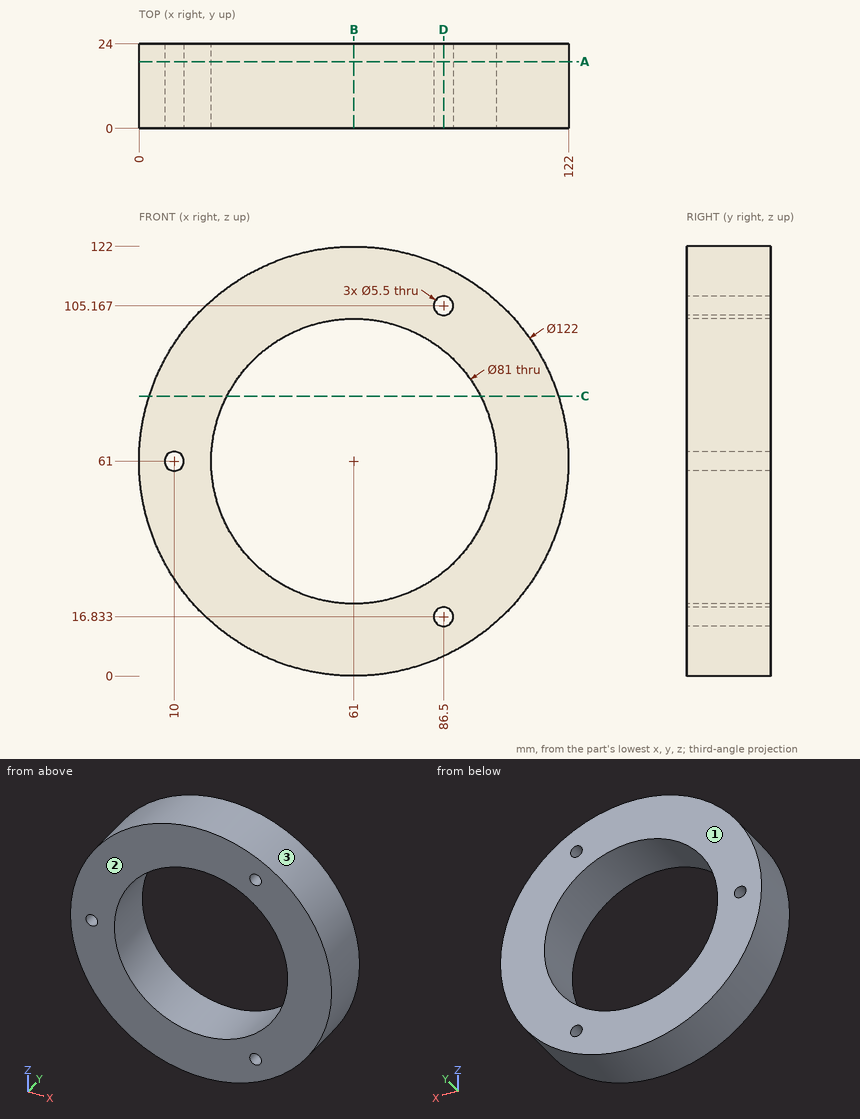
Study the drawing (mm; zero at the part's minimum x, y, z) and answer. Round coordinates to 2 decimals unless told otherwise and drop trailing zeros. Loops run counter-clockwise (first coordinate to the right, second up) from the corner with the lowest first, then second, coordinate; pieces in that order, holes last.
Q1. Given pin 1 Ø1.5 at (x, y) = (14, 12.5) entering from -Z; pin 2 Ø3 at (y, z) = (4.5, 54.5) entering from +X (1 decimal); pin 3 Ø6 at (y, z) = (3.5, 24.5) entering from +X; pin 4 Ø3.5 at (x, z) = (86.5, 16.83) entering from +Y, each flat-ended and moving along its own axis, determine where each tip first touches the part or whether it passes through.
Q2. Section B-B, the plane x = 61 is taken. Determine the outline of the cut face in (y, z), then the cut area to 3 significant figures.
Q3. Section D-D, the plane x = 86.5 is taken. Determine the outline of the cut face in (y, z).
Q4. Find the intervals of material crossed by line 1 (Z direction, x = 60.5, y = 4.5); line 2 (Z direction, x = 86.5, y = 6) (1 decimal); line 3 (Z direction, x = 40.5, y = 6.25), in increasing order.
Q5. For a pull along Y with two mould halves and no side action, classify the marked faces 1, 2 and 3 as released by +Y, released by -Y, zero draft, split by the parting line, or undercut.
Q6. Section A-A, the plane y = 19 is taken. Determine the outline of the cut face in (x, z).
Q7. Section C-C, the plane z = 79.5 is taken. Determine the outline of the cut face in (x, y).
Completed:
1. pin 1: stops at z = 21.23
1. pin 2: stops at x = 121.8
1. pin 3: stops at x = 111.98
1. pin 4: passes through
2. outline: (0, 0) - (24, 0) - (24, 20.5) - (0, 20.5) - close; (0, 101.5) - (24, 101.5) - (24, 122) - (0, 122) - close
2. area: 984 mm2
3. outline: (0, 5.59) - (24, 5.59) - (24, 14.08) - (0, 14.08) - close; (0, 19.58) - (24, 19.58) - (24, 29.54) - (0, 29.54) - close; (0, 92.46) - (24, 92.46) - (24, 102.42) - (0, 102.42) - close; (0, 107.92) - (24, 107.92) - (24, 116.41) - (0, 116.41) - close
4. line 1: z = 0 to 20.5, 101.5 to 122
4. line 2: z = 5.6 to 14.1, 19.6 to 29.5, 92.5 to 102.4, 107.9 to 116.4
4. line 3: z = 3.55 to 26.07, 95.93 to 118.45
5. face 1: released by +Y
5. face 2: released by -Y
5. face 3: zero draft
6. outline: circle Ø122 at (61, 61); hole circle Ø5.5 at (10, 61); hole circle Ø81 at (61, 61); hole circle Ø5.5 at (86.5, 16.83); hole circle Ø5.5 at (86.5, 105.17)
7. outline: (2.87, 0) - (24.97, 0) - (24.97, 24) - (2.87, 24) - close; (97.03, 0) - (119.13, 0) - (119.13, 24) - (97.03, 24) - close
